Design review of the part built by this model. Coordinates are the model's own, in mm. A direction names the side the tool comes from. Round coordinates to 2 decimals unless told otherwise and drop trailing zeros. Order: outer loops, then holes, each group sorted by start corner. A loop starts at its lowest first (then second) coordinate and runs counter-clockwise, first axis right, second up. Notation, with made-up numbers: M 55,-0.75 L 109,-0.75 A32 cw 109,35.25 Z; hole C 67,0.5 d8. An arc over 180 degrees is marked long. Write each question's results on one line, items separated by ' | '. Start each with the question number.
Item 1: Wall thickness on line 1 (X direction, y = -143.5, z = -1); line 2 (Z direction, x = -17, y = -20): over which ranges is each line inside the solid? List them lowest first. Write a range as [from, to].
Item 2: The part is to be moulded in two halves that separate along X. For faces 3 (the flat face through (-18.35, -986, 0)), 4 (the flat face through (0, 0, -16)), 5 (the flat face through (15.35, -986, 0)), say which applies: +X half, -X half, draft (parallel to the pull), parting line (faces both ways), or undercut.
Item 3: Clearance check with flat-ended pins moving along their axes: pin 1 (15.5 mm diameter, centred on x = -1.5, y = -640, fed in from +Z); pin 2 (4 mm diameter, centred on x = 0.5, y = -534.5, fed in from +Z). State where each tip first meets the part, or that it passes through.
Item 4: Take a section at A-A, the plane z = 0. Write out the cut boundary in (x, y).
Item 5: Machinability: for faces 1 (the flat face through (0, -986, -18.35)), 2 (the flat face through (-15.35, -986, 0)), which of the approach directions +Z, -Z, +X, -X, +Y, -Y give a long, thin tool a straight path to every point of the face, cutting with its end or side? Answer none if there is none.
Item 6: Take a section at B-B, the plane y = -1218. Write out the cut boundary in (x, z), plus the area to 3 significant figures.
```python
from build123d import *

# Parameters (mm, degrees)
F1_DEPTH = 2000
F2_R     = 8
F3_DEPTH = 36.701


with BuildPart() as f1:
    # F0 (on Front) → F1 (new body)
    with BuildSketch(Plane.XZ):
        with BuildLine():
            Line((15.35, 15.35), (15.35, -15.35))
            Line((15.35, -15.35), (-15.35, -15.35))
            Line((-15.35, -15.35), (-15.35, 15.35))
            Line((-15.35, 15.35), (-9, 15.35))
            Line((-9, 15.35), (-9, 18.35))
            Line((-9, 18.35), (-16.85, 18.35))
            ThreePointArc((-16.85, 18.35), (-17.91066, 17.91066), (-18.35, 16.85))
            Line((-18.35, 16.85), (-18.35, -16.85))
            ThreePointArc((-18.35, -16.85), (-17.91066, -17.91066), (-16.85, -18.35))
            Line((-16.85, -18.35), (16.85, -18.35))
            ThreePointArc((16.85, -18.35), (17.91066, -17.91066), (18.35, -16.85))
            Line((18.35, -16.85), (18.35, 16.85))
            ThreePointArc((18.35, 16.85), (17.91066, 17.91066), (16.85, 18.35))
            Line((16.85, 18.35), (9, 18.35))
            Line((9, 18.35), (9, 15.35))
            Line((9, 15.35), (15.35, 15.35))
        make_face()
    extrude(amount=F1_DEPTH)

    # F2 (on face) → F3 (cut, through all)
    with BuildSketch(Plane.YZ.offset(18.35)):
        with Locations((-20, 0)):
            Circle(F2_R)
    extrude(amount=-F3_DEPTH, mode=Mode.SUBTRACT)


solid = f1.part
```
Results list:
1) line 1: [-18.35, -15.35], [15.35, 18.35] | line 2: [-18.34, -8], [8, 18.34]
2) face 3: -X half | face 4: draft | face 5: undercut
3) pin 1: z = 18.35 | pin 2: z = -15.35
4) outline: M -18.35,-2000 L -15.35,-2000 L -15.35,-28 L -18.35,-28 Z; M -18.35,-12 L -15.35,-12 L -15.35,0 L -18.35,0 Z; M 15.35,-2000 L 18.35,-2000 L 18.35,-28 L 15.35,-28 Z; M 15.35,-12 L 18.35,-12 L 18.35,0 L 15.35,0 Z
5) face 1: -Z, +X, -X, +Y, -Y | face 2: +Y, -Y
6) outline: M -18.35,-16.85 A1.5 ccw -16.85,-18.35 L 16.85,-18.35 A1.5 ccw 18.35,-16.85 L 18.35,16.85 A1.5 ccw 16.85,18.35 L 9,18.35 L 9,15.35 L 15.35,15.35 L 15.35,-15.35 L -15.35,-15.35 L -15.35,15.35 L -9,15.35 L -9,18.35 L -16.85,18.35 A1.5 ccw -18.35,16.85 Z | area: 348 mm²
